Build history of the part. All positions in model axes, mm. Coordinates: 2 decimals unless noted, no trailing zeros. Order: outer loops, then holes, each group sorted by start corner. A loop starts at its lowest first (then second) coordinate and runs counter-clockwise, first axis right, second up. Notation, with made-up numbers: (84, 80) -> (129, 80) arc R31 ccw to (129, 106) -> close; hole circle Ø7 at (51.5, -19.5). An arc over 180 degrees is marked (long way). Write each question's results on one line, items separated by ' | '.
from build123d import *

# Parameters (mm, degrees)
SKETCH1_R           = 2
SKETCH1_R_2         = 5
BOSS_EXTRUDE2_DEPTH = 3


with BuildPart() as part:
    # Sketch1 → Boss-Extrude2 (new body)
    # profile 1 of 2: a face of its own
    with BuildSketch(Plane(origin=(0, 0, 0), x_dir=(1, 0, 0), z_dir=(0, 1, 0))):
        with BuildLine():
            Line((-36.606010435, -62), (0, -62))
            Line((0, -62), (21, -62))
            Line((21, -62), (21, -61))
            ThreePointArc((21, -61), (19, -59), (21, -57))
            Line((21, -57), (21, -39))
            ThreePointArc((21, -39), (19, -37), (21, -35))
            Line((21, -35), (21, 35))
            ThreePointArc((21, 35), (19, 37), (21, 39))
            Line((21, 39), (21, 57))
            ThreePointArc((21, 57), (19, 59), (21, 61))
            Line((21, 61), (21, 62))
            Line((21, 62), (-36.606010435, 62))
            ThreePointArc((-36.606010435, 62), (-72, 0), (-36.606010435, -62))
        make_face()
        with Locations(Location((-65, -15, 0), (0, 0, 270))):
            Circle(SKETCH1_R, mode=Mode.SUBTRACT)
        with Locations(Location((-40, -15, 0), (0, 0, 270))):
            Circle(SKETCH1_R, mode=Mode.SUBTRACT)
        with Locations(Location((-25.455844123, -25.455844123, 0), (0, 0, 270))):
            Circle(SKETCH1_R, mode=Mode.SUBTRACT)
        with Locations(Location((0, -34, 0), (0, 0, 270))):
            Circle(SKETCH1_R_2, mode=Mode.SUBTRACT)
        with Locations(Location((-65, 15, 0), (0, 0, 270))):
            Circle(SKETCH1_R, mode=Mode.SUBTRACT)
        with Locations(Location((-40, 15, 0), (0, 0, 270))):
            Circle(SKETCH1_R, mode=Mode.SUBTRACT)
        with Locations(Location((-25.455844123, 25.455844123, 0), (0, 0, 270))):
            Circle(SKETCH1_R, mode=Mode.SUBTRACT)
        with Locations(Location((0, 34, 0), (0, 0, 270))):
            Circle(SKETCH1_R_2, mode=Mode.SUBTRACT)
    # profile 2 of 2: a face of its own
    with BuildSketch(Plane(origin=(0, 0, 0), x_dir=(1, 0, 0), z_dir=(0, 1, 0))):
        with BuildLine():
            Line((21, -62), (36.606010435, -62))
            ThreePointArc((36.606010435, -62), (62.528524496, -35.695708766), (72, 0))
            ThreePointArc((72, 0), (62.528524496, 35.695708766), (36.606010435, 62))
            Line((36.606010435, 62), (21, 62))
            Line((21, 62), (21, 61))
            ThreePointArc((21, 61), (22.414213562, 60.414213562), (23, 59))
            ThreePointArc((23, 59), (22.414213562, 57.585786438), (21, 57))
            Line((21, 57), (21, 39))
            ThreePointArc((21, 39), (22.414213562, 38.414213562), (23, 37))
            ThreePointArc((23, 37), (22.414213562, 35.585786438), (21, 35))
            Line((21, 35), (21, -35))
            ThreePointArc((21, -35), (22.414213562, -35.585786438), (23, -37))
            ThreePointArc((23, -37), (22.414213562, -38.414213562), (21, -39))
            Line((21, -39), (21, -57))
            ThreePointArc((21, -57), (22.414213562, -57.585786438), (23, -59))
            ThreePointArc((23, -59), (22.414213562, -60.414213562), (21, -61))
            Line((21, -61), (21, -62))
        make_face()
        with Locations(Location((25.455844123, -25.455844123, 0), (0, 0, 270))):
            Circle(SKETCH1_R, mode=Mode.SUBTRACT)
        with Locations(Location((40, -15, 0), (0, 0, 270))):
            Circle(SKETCH1_R, mode=Mode.SUBTRACT)
        with Locations(Location((65, -15, 0), (0, 0, 270))):
            Circle(SKETCH1_R, mode=Mode.SUBTRACT)
        with Locations(Location((25.455844123, 25.455844123, 0), (0, 0, 270))):
            Circle(SKETCH1_R, mode=Mode.SUBTRACT)
        with Locations(Location((40, 15, 0), (0, 0, 270))):
            Circle(SKETCH1_R, mode=Mode.SUBTRACT)
        with Locations(Location((65, 15, 0), (0, 0, 270))):
            Circle(SKETCH1_R, mode=Mode.SUBTRACT)
    extrude(amount=BOSS_EXTRUDE2_DEPTH)


solid = part.part
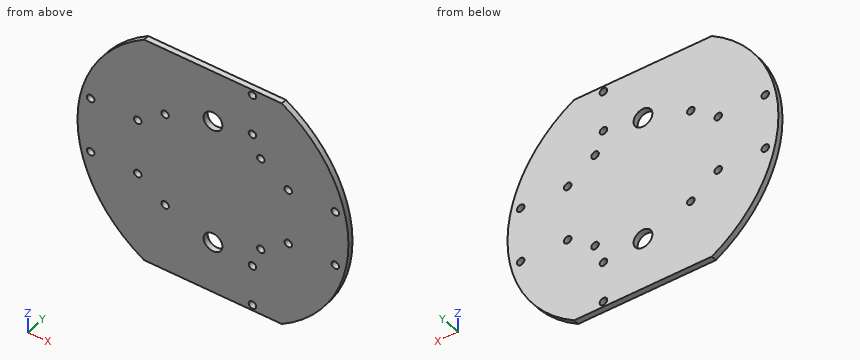
Item 1: Pin check, flat tips, straight feed: pin 1 (3 mm diameter, centred on x = -65, z = 15, fed in from +Y); pin 2 (4.5 mm diameter, centred on x = -40, z = 15, fed in from -Y); pin 3 (1 mm diameter, centred on y = 2.5, z = -49.5, fed in from +X); pin 4 (1.5 mm diameter, centred on x = 57, y = 0.5, fed in from +Z). Stop position of each tip, or through.
Answer:
pin 1: passes through | pin 2: stops at y = 0 | pin 3: stops at x = 52.75 | pin 4: stops at z = 44.94
Item 2: Drill centre lines: line 1 (X direction, y = 1.25, z = 27); line 2 (Z direction, x = 38.5, y = 0.7); line 3 (Z direction, x = -1, y = 1.1). Where is each one in solid material? Low to high. Write a range as from..to.
Answer:
line 1: x = -66.75..-26.73, -24.18..24.18, 26.73..66.75 | line 2: z = -60.84..-16.32, -13.68..13.68, 16.32..60.84 | line 3: z = -62..-38.9, -29.1..29.1, 38.9..62
Item 3: Slice it at D-D, the plane z = -15. List the corners of the cut face in (x, y).
Answer:
outline: (-70.42, 0) -> (-67, 0) -> (-67, 3) -> (-70.42, 3) -> close; (-63, 0) -> (-42, 0) -> (-42, 3) -> (-63, 3) -> close; (-38, 0) -> (38, 0) -> (38, 3) -> (-38, 3) -> close; (42, 0) -> (63, 0) -> (63, 3) -> (42, 3) -> close; (67, 0) -> (70.42, 0) -> (70.42, 3) -> (67, 3) -> close
Item 4: Slice it at A-A, the plane z = 25. List the corners of the cut face in (x, y).
Answer:
outline: (-67.52, 0) -> (-27.4, 0) -> (-27.4, 3) -> (-67.52, 3) -> close; (-23.51, 0) -> (23.51, 0) -> (23.51, 3) -> (-23.51, 3) -> close; (27.4, 0) -> (67.52, 0) -> (67.52, 3) -> (27.4, 3) -> close
Item 5: Slice it at C-C, the plane y = 1.4. State how many separate pieces and enclosed holes the cut face has, and give its area (3 significant figures).
Answer:
separate pieces: 1 | enclosed holes: 18 | area: 14,900 mm^2
Item 6: Slice it at B-B, the plane x = 40. List the corners of the cut face in (y, z).
Answer:
outline: (0, -59.87) -> (3, -59.87) -> (3, -17) -> (0, -17) -> close; (0, -13) -> (3, -13) -> (3, 13) -> (0, 13) -> close; (0, 17) -> (3, 17) -> (3, 59.87) -> (0, 59.87) -> close
